For this review, take the finished solid that the model builds, in its own axes (mm). Face numbers are marked on the shaded views. A direction names the side the tool comes from. Coordinates: 2 decimals unless noted, no trailing zeros. Order: outer loops, then holes, each group sorted by start corner. A loop starts at its lowest first (then second) coordinate and runs counter-clockwise, first axis right, second up. Notation, with made-up numbers: (54.25, 52) - (107.25, 52) arc R9 cw to (107.25, 62) - close; hole circle Ø6 at (1.5, -20). An arc over 180 degrees is marked (long way). One line per item, written item: value. Start each with the question number.
(1) To check wall thickness, follow line 1 along Z through (x, y) = (-3, 0.5); line 2 along Z through (x, y) = (-0.5, -1.5); line 3 along Y through (x, z) = (0, -2.75). State the ranges of each line that lie inside material, in increasing order.
(2) Consider section A-A on y = 0. Write out the cut boundary in (x, z).
(3) Clearance check with flat-ended pins moving along their axes: pin 1 (1 mm diameter, centred on x = 2, z = 4.5, fed in from -Y); pin 2 (3 mm diameter, centred on x = 2, z = -3, fed in from -Y); pin 3 (1.5 mm diameter, centred on y = 0, z = 0, fed in from +X). State where each tip first meets the part, or that it passes through.
(4) For the marked faces 1, 2 and 3, list the 3-axis set-ups (+Z, -Z, +X, -X, +Y, -Y) from which the entire face can be reached by the end or side of a thin tool; tool diameter is ignored.
(5) Consider section D-D on y = -1.25. Write out the cut boundary in (x, z).
(6) Consider section C-C on z = -1.25. Write out the cut boundary in (x, y), then the cut area to 3 significant figures.
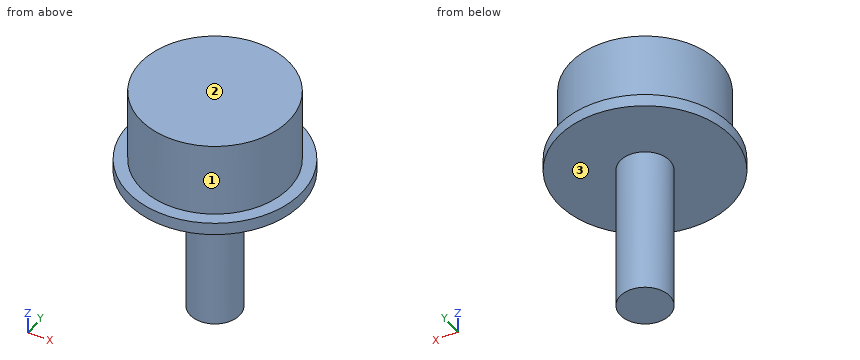
```python
from build123d import *


with BuildPart() as part:
    # Skizze1 → Rotation1 (revolve)
    with BuildSketch(Plane(origin=(0, 0, 0), x_dir=(0, 0, -1), z_dir=(1, 0, 0))):
        Polygon((4, 1), (4, 0), (-4, 0), (-3, 1), align=None)
    revolve(axis=Axis((0, 0, 0), (0, 0, 1)))

    # Skizze2 → Rotation2 (revolve)
    with BuildSketch(Plane(origin=(0, 0, 0), x_dir=(0, 0, -1), z_dir=(1, 0, 0))):
        Polygon((-2.5, 3), (-5.5, 3), (-5.5, 0), (-2, 0), (-2, 3.5), (-2.5, 3.5), align=None)
    revolve(axis=Axis((0, 0, 2), (0, 0, -1)))


solid = part.part
```
Geometry check:
1. line 1: z = 2 to 2.5
1. line 2: z = 2 to 5.5
1. line 3: y = -1 to 1
2. outline: (-3.5, 2) - (-1, 2) - (-1, -4) - (1, -4) - (1, 2) - (3.5, 2) - (3.5, 2.5) - (3, 2.5) - (3, 5.5) - (-3, 5.5) - (-3, 2.5) - (-3.5, 2.5) - close
3. pin 1: stops at y = -2.6
3. pin 2: stops at y = -0.87
3. pin 3: stops at x = 1
4. face 1: +Z
4. face 2: +Z, +X, -X, +Y, -Y
4. face 3: -Z
5. outline: (-3.27, 2) - (3.27, 2) - (3.27, 2.5) - (2.73, 2.5) - (2.73, 5.5) - (-2.73, 5.5) - (-2.73, 2.5) - (-3.27, 2.5) - close
6. outline: circle Ø2 at (0, 0)
6. area: 3.14 mm^2
